Verification items for this drawing (mm, ordinates from the low corner). Round coordinates to 2 decimals unless told otherwise and drop trailing zeros. Write each loop counter-clockwise with the first axis right and the second up, starting at its lowest first coordinate (ties: lowest second). Pieces come first, ordered by that corner, then holes.
Item 1: Cross-section at A-A (z = 4.46). Enter the section's corners in (x, y).
Item 2: Depth check by flat-ended pin: P1, Ø3, axis at x = 5.5, z = 40.5, coming from the +Y side; P2, Ø0.8, axis at y = 4.5, z = 44.5, coming from the -X side; P3, Ø0.5, axis at x = 6.5, z = 47, coming from the +Y side. Enter the tip coordinate at first touch or a pass-through.
Item 3: Cross-section at C-C (z = 38). Enter the section's corners in (x, y).
Item 4: Cross-section at D-D (z = 67). Enter the section's corners in (x, y), then the cut area to 3 significant figures.
Item 5: Cross-section at B-B (y = 1.9). Enter the section's corners in (x, z).
Item 6: Scan lines: probe 1 along Z at (x, y) = (4.25, 3.05); probe 2 along Z at (x, y) = (3.75, 1.55); probe 3 along Z at (x, y) = (1.25, 1). Record each from-to range of solid material in increasing order.
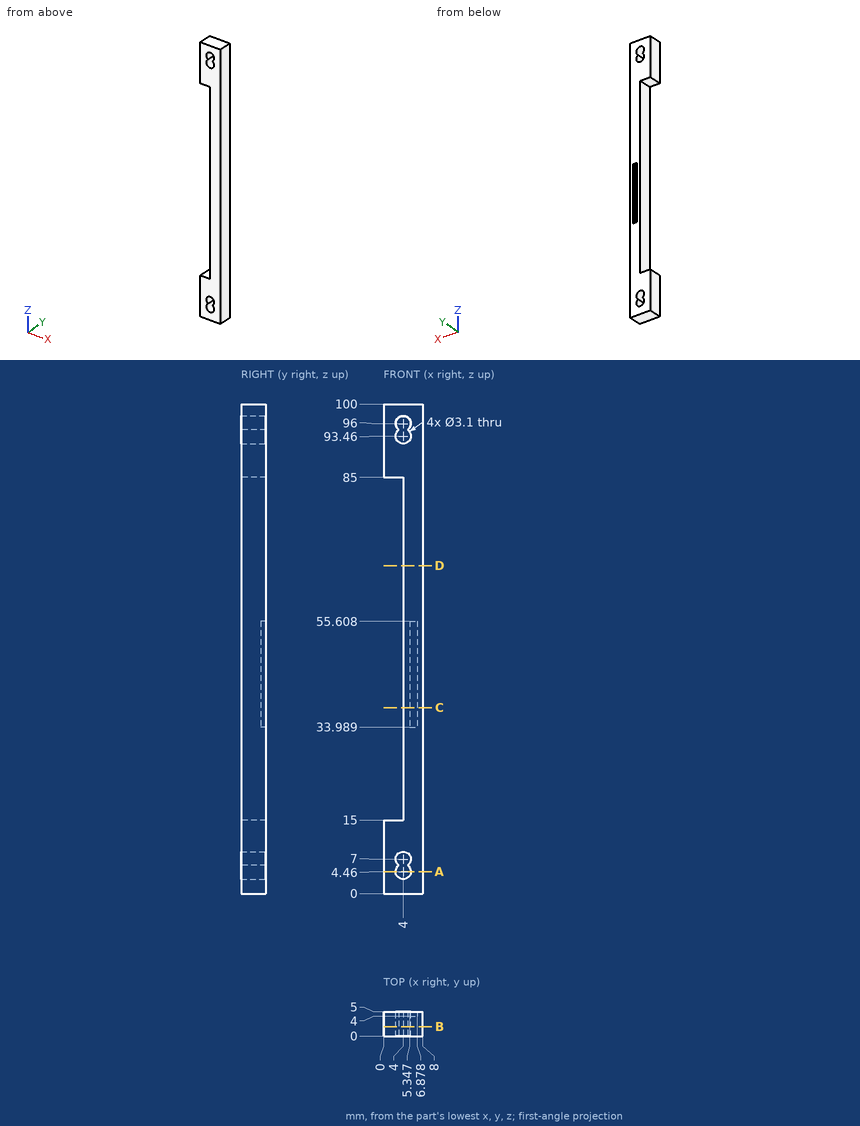
Resolved:
1. outline: (0, 0) - (2.45, 0) - (2.45, 5) - (0, 5) - close; (5.55, 0) - (8, 0) - (8, 5) - (5.55, 5) - close
2. P1: stops at y = 5
2. P2: stops at x = 4
2. P3: stops at y = 4
3. outline: (4, 0) - (8, 0) - (8, 5) - (6.88, 5) - (6.88, 4) - (5.35, 4) - (5.35, 5) - (4, 5) - close
4. outline: (4, 0) - (8, 0) - (8, 5) - (4, 5) - close
4. area: 20.0 mm2
5. outline: (0, 0) - (8, 0) - (8, 100) - (0, 100) - (0, 85) - (4, 85) - (4, 15) - (0, 15) - close; hole (3.11, 5.73) arc R1.55 ccw (long way) to (4.89, 5.73) arc R1.55 ccw (long way) to start; hole (3.11, 94.73) arc R1.55 ccw (long way) to (4.89, 94.73) arc R1.55 ccw (long way) to start
6. probe 1: z = 0 to 2.93, 8.53 to 91.93, 97.53 to 100
6. probe 2: z = 0 to 2.93, 8.53 to 15, 85 to 91.93, 97.53 to 100
6. probe 3: z = 0 to 15, 85 to 100
